```python
from build123d import *

# Parameters (mm, degrees)
SKETCH1_W               = 605.082945164
SKETCH1_H               = 1243.943840666
BOSS_EXTRUDE1_DEPTH     = 2.54
SKETCH3_R               = 72.07245037
SKETCH3_R_2             = 37.854305462
CUT_EXTRUDE1_DEPTH      = 1
CUT_EXTRUDE1_DEPTH_BACK = 3.54


with BuildPart() as part:
    # Sketch1 → Boss-Extrude1 (new body)
    with BuildSketch(Plane.XY):
        with Locations((-316.280332246, 820.569825563)):
            Rectangle(SKETCH1_W, SKETCH1_H)
    extrude(amount=BOSS_EXTRUDE1_DEPTH)

    # Sketch3 → Cut-Extrude1 (cut, two sides)
    with BuildSketch(Plane.XY.offset(2.54)) as cut_extrude1_sk:
        with Locations((-520.126168734, 1312.226670832)):
            Circle(SKETCH3_R)
        with Locations((-151.601482637, 581.817383071)):
            Circle(SKETCH3_R_2)
    extrude(amount=CUT_EXTRUDE1_DEPTH, mode=Mode.SUBTRACT)
    extrude(cut_extrude1_sk.sketch, amount=-CUT_EXTRUDE1_DEPTH_BACK, mode=Mode.SUBTRACT)


solid = part.part
```
Design review of the part built by this model. Coordinates are the model's own, in mm. Round coordinates to 2 decimals unless told otherwise and drop trailing zeros. Order: outer loops, then holes, each group sorted by start corner. A loop starts at its lowest first (then second) coordinate and runs counter-clockwise, first axis right, second up. Notation, with made-up numbers: (-1, 35) - (34, 35) arc R6 ccw to (34, 45) - close; hole circle Ø3 at (28, -26). An arc over 180 degrees is marked (long way). Return JSON: item names as keys, results as strings.
Q1. Consider section A-A on x = -562. Write out the cut boundary in (y, z).
Computed values:
{"outline": "(198.6, 0) - (1253.57, 0) - (1253.57, 2.54) - (198.6, 2.54) - close; (1370.89, 0) - (1442.54, 0) - (1442.54, 2.54) - (1370.89, 2.54) - close"}
Q2. The part is to be moulded in two halves that separate along Y. For faces 1 (the cylindrical face through (-179.5, 607.4, 1.3)), 2 (the flat face through (-321, 829, 0)), 3 (the cylindrical face through (-486.869, 1248.286, 1.288)), say which applies: pulls with the +Y half, pulls with the -Y half, needs draft (parallel to the pull), parting line crosses it, or undercut.
Computed values:
{"face 1": "undercut", "face 2": "needs draft", "face 3": "undercut"}
Q3. Consider section B-B on y = 1262.5. Write out the cut boundary in (x, z), plus the area to 3 significant figures.
Computed values:
{"outline": "(-618.82, 0) - (-572.3, 0) - (-572.3, 2.54) - (-618.82, 2.54) - close; (-467.96, 0) - (-13.74, 0) - (-13.74, 2.54) - (-467.96, 2.54) - close", "area": "1,270 mm2"}
Q4. Consider section C-C on z = 0.6. Write out the cut boundary in (x, y), plus the area to 3 significant figures.
Computed values:
{"outline": "(-618.82, 198.6) - (-13.74, 198.6) - (-13.74, 1442.54) - (-618.82, 1442.54) - close; hole circle Ø144.14 at (-520.13, 1312.23); hole circle Ø75.71 at (-151.6, 581.82)", "area": "732,000 mm2"}
Q5. Wall thickness on L1, parallel to X at y = 580, z = 0.4; L2, parallel to Y at x = -186.5, z = 2.05; L3, parallel to X at y = 1256, z = 1.3: over which ranges is each line inside the solid? List them lowest first. Write a range as [from, to].
Computed values:
{"L1": "x = [-618.82, -189.41], [-113.79, -13.74]", "L2": "y = [198.6, 567.15], [596.48, 1442.54]", "L3": "x = [-618.82, -565.21], [-475.04, -13.74]"}
